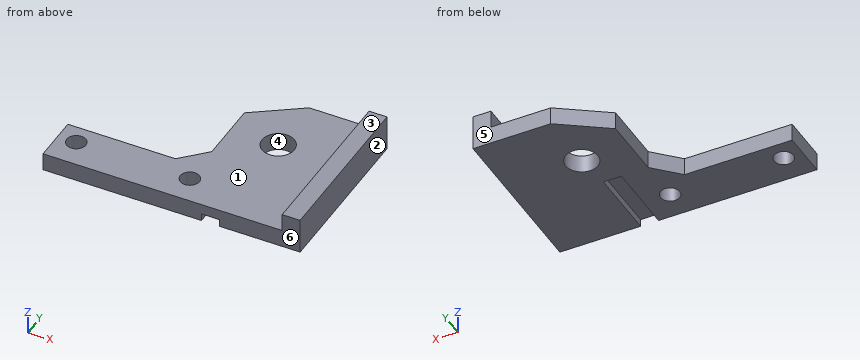
```python
from build123d import *

# Parameters (mm, degrees)
SKETCH1_R           = 1.6
SKETCH1_R_2         = 2.7
BOSS_EXTRUDE1_DEPTH = 3
BOSS_EXTRUDE2_START = 3
SKETCH1_3_W         = 3
SKETCH1_3_H         = 28
BOSS_EXTRUDE2_DEPTH = 3
SKETCH1_5_W         = 3
SKETCH1_5_H         = 12
CUT_EXTRUDE2_DEPTH  = 1.25


with BuildPart() as part:
    # Sketch1 → Boss-Extrude1 (new body)
    with BuildSketch(Plane.XY):
        Polygon((0, 0), (0, 28), (-13, 28), (-21, 22.5), (-21, 12), (-25, 8), (-43, 8), (-43, 0), align=None)
        with Locations((-39.9, 4.75)):
            Circle(SKETCH1_R, mode=Mode.SUBTRACT)
        with Locations((-13, 18)):
            Circle(SKETCH1_R_2, mode=Mode.SUBTRACT)
        with Locations((-20.9, 4.75)):
            Circle(SKETCH1_R, mode=Mode.SUBTRACT)
    extrude(amount=BOSS_EXTRUDE1_DEPTH)

    # Sketch1<3> → Boss-Extrude2 (add)
    with BuildSketch(Plane.XY.offset(BOSS_EXTRUDE2_START)):
        with Locations((-1.5, 14)):
            Rectangle(SKETCH1_3_W, SKETCH1_3_H)
    extrude(amount=BOSS_EXTRUDE2_DEPTH)

    # Sketch1<5> → Cut-Extrude2 (cut)
    with BuildSketch(Plane.XY):
        with Locations((-15, 6)):
            Rectangle(SKETCH1_5_W, SKETCH1_5_H)
    extrude(amount=CUT_EXTRUDE2_DEPTH, mode=Mode.SUBTRACT)


solid = part.part
```
Model file for the job. Use its own axes, mm. Face numbers are marked on the shaded views. A direction names the side the tool comes from. Give positions to 0.01 mm unless a question says otherwise; leave off trailing zeros. Order: outer loops, then holes, each group sorted by start corner. A loop starts at its lowest first (then second) coordinate and runs counter-clockwise, first axis right, second up.
1) Saw through at C-C, the plane z = 2.1. Write the cut outline in (x, y).
2) Pin check, flat tips, straight feed: pin 1 (2.5 mm diameter, centred on y = 16.5, z = 2, fed in from -X); pin 2 (2.5 mm diameter, centred on x = -38, z = 1.5, fed in from +Y); pin 3 (3.5 mm diameter, centred on x = -14.5, y = 3.5, fed in from -Z); pin 4 (5 mm diameter, centred on x = -39.9, y = 4.75, fed in from +Z). Stop position of each tip, or through.
3) 3-axis set-ups, long thin cutter, end or side, ignore diameter. For the marked faces 1 and 2: which of +Z, -Z, +X, -X, +Y, -Y reach the whole face in a straight line?
4) Wall check: probe 1 along Y at (x, z) = (-39.9, 1.95); probe 2 along X at (y, z) = (5.5, 1.2); probe 3 along Y at (x, z) = (-37, 2.4). Give the ranges that are in metal, low to high.
5) Saw through at B-B, the plane x = -39.9. Write the cut outline in (y, z), then the cut area to 3 significant figures.
6) Saw through at D-D, the plane y = 10.5. Write the cut outline in (x, z), then the cut area to 4 significant figures.
7) Saw through at A-A, the plane y = 18. Write the cut outline in (x, z).
8) Mould opens along Y. For the marked faces 3, 4, 5 and 6 say: +Y half, -Y half, draft (parallel to the pull), parting line (faces both ways), or undercut.
Computed:
1. outline: (-43, 0) - (0, 0) - (0, 28) - (-13, 28) - (-21, 22.5) - (-21, 12) - (-25, 8) - (-43, 8) - close; hole circle Ø3.2 at (-39.9, 4.75); hole circle Ø3.2 at (-20.9, 4.75); hole circle Ø5.4 at (-13, 18)
2. pin 1: stops at x = -21
2. pin 2: stops at y = 8
2. pin 3: stops at z = 0
2. pin 4: stops at z = 3
3. face 1: +Z, -X, +Y, -Y
3. face 2: +Z, -Z, +X, +Y, -Y
4. probe 1: y = 0 to 3.15, 6.35 to 8
4. probe 2: x = -43 to -41.31, -38.49 to -22.31, -19.49 to -16.5, -13.5 to 0
4. probe 3: y = 0 to 8
5. outline: (0, 0) - (3.15, 0) - (3.15, 3) - (0, 3) - close; (6.35, 0) - (8, 0) - (8, 3) - (6.35, 3) - close
5. area: 14.4 mm2
6. outline: (-22.5, 0) - (-16.5, 0) - (-16.5, 1.25) - (-13.5, 1.25) - (-13.5, 0) - (0, 0) - (0, 6) - (-3, 6) - (-3, 3) - (-22.5, 3) - close
6. area: 72.75 mm2
7. outline: (-21, 0) - (-15.7, 0) - (-15.7, 3) - (-21, 3) - close; (-10.3, 0) - (0, 0) - (0, 6) - (-3, 6) - (-3, 3) - (-10.3, 3) - close
8. face 3: draft
8. face 4: undercut
8. face 5: +Y half
8. face 6: -Y half
